Geometry check sheet. Reference: the model listing, model coordinates, mm. A direction names the side the tool comes from. Give positions to 0.01 mm unless a question says otherwise; leave off trailing zeros. Order: outer loops, then holes, each group sorted by start corner. A loop starts at its lowest first (then second) coordinate and runs counter-clockwise, first axis right, second up. Notation, with made-up numbers: M -20,-37.5 L -14,-37.5 A23 ccw -14,-23.5 Z; hole C -38.75,40.5 d11. An arc over 180 degrees is marked long. Answer as CSV lines item,"result".
from build123d import *

# Parameters (mm, degrees)
SKETCH4_R           = 6
BOSS_EXTRUDE3_DEPTH = 1
SKETCH5_R           = 5
SKETCH5_R_2         = 4
BOSS_EXTRUDE4_DEPTH = 4.75
CUT_EXTRUDE3_START  = -3
SKETCH9_R           = 4
CUT_EXTRUDE3_DEPTH  = 3
CUT_EXTRUDE7_DEPTH  = 10
CUT_EXTRUDE8_DEPTH  = 10
CUT_EXTRUDE10_START = -6
CUT_EXTRUDE10_DEPTH = 6
SKETCH14_R          = 2.4
CUT_EXTRUDE11_DEPTH = 6


with BuildPart() as part:
    # Sketch4 → Boss-Extrude3 (new body)
    with BuildSketch(Plane(origin=(0, 0, 0), x_dir=(1, 0, 0), z_dir=(0, 1, 0))):
        with Locations(Location((0, 0, 0), (0, 0, 270))):
            Circle(SKETCH4_R)
    extrude(amount=BOSS_EXTRUDE3_DEPTH)

    # Sketch5 → Boss-Extrude4 (add)
    with BuildSketch(Plane(origin=(0, 1, 0), x_dir=(1, 0, 0), z_dir=(0, 1, 0))):
        with Locations(Location((0, 0, 0), (0, 0, 270))):
            Circle(SKETCH5_R)
        with Locations(Location((0, 0, 0), (0, 0, 270))):
            Circle(SKETCH5_R_2, mode=Mode.SUBTRACT)
    extrude(amount=BOSS_EXTRUDE4_DEPTH)

    # Sketch6 → Revolve4 (revolve)
    with BuildSketch(Plane.XY, mode=Mode.PRIVATE) as revolve4_sk:
        Polygon((0, 5.75), (5, 5.75), (6, 7), (0, 7), align=None)
    revolve(revolve4_sk.sketch.rotate(Axis((0, 5.75, 0), (0, 1, 0)), 270), axis=Axis((0, 5.75, 0), (0, 1, 0)))

    # Sketch9 → Cut-Extrude3 (cut)
    with BuildSketch(Plane(origin=(0, 7, 0), x_dir=(1, 0, 0), z_dir=(0, 1, 0)).offset(CUT_EXTRUDE3_START)):
        with Locations(Location((0, 0, 0), (0, 0, 270))):
            Circle(SKETCH9_R)
    extrude(amount=CUT_EXTRUDE3_DEPTH, mode=Mode.SUBTRACT)

    # Sketch11 → Cut-Extrude7 (cut)
    with BuildSketch(Plane.XY):
        Polygon((0, 4.575), (0, 3.375), (1.2, 3.375), (1.6, 3.375), align=None)
        Polygon((-1.2, 3.375), (0, 3.375), (0, 4.575), (-1.6, 3.375), align=None)
        Polygon((0, 2.175), (0, 3.375), (-1.2, 3.375), (-1.6, 3.375), align=None)
        Polygon((1.2, 3.375), (0, 3.375), (0, 2.175), (1.6, 3.375), align=None)
    extrude(amount=CUT_EXTRUDE7_DEPTH, mode=Mode.SUBTRACT)

    # Sketch12 → Cut-Extrude8 (cut)
    with BuildSketch(Plane(origin=(0, 0, 0), x_dir=(0, 0, -1), z_dir=(1, 0, 0))):
        with BuildLine():
            ThreePointArc((0.6, 3.375), (0.424264069, 3.799264069), (0, 3.975))
            Line((0, 3.975), (0, 2.775))
            ThreePointArc((0, 2.775), (0.424264069, 2.950735931), (0.6, 3.375))
        make_face()
        with BuildLine():
            Line((0, 2.775), (0, 3.975))
            ThreePointArc((0, 3.975), (-0.6, 3.375), (0, 2.775))
        make_face()
    extrude(amount=CUT_EXTRUDE8_DEPTH, mode=Mode.SUBTRACT)

    # Sketch13 → Cut-Extrude10 (cut)
    with BuildSketch(Plane(origin=(0, 7, 0), x_dir=(1, 0, 0), z_dir=(0, 1, 0)).offset(CUT_EXTRUDE10_START)):
        with BuildLine():
            Line((-4.779206309, -3.627559381), (-3.72991173, -1.444907777))
            ThreePointArc((-3.72991173, -1.444907777), (-3.947043415, 0.648728201), (-3.071224525, 2.562728998))
            Line((-3.071224525, 2.562728998), (-4.606836788, 3.844093497))
            ThreePointArc((-4.606836788, 3.844093497), (-5.99840399, 0.138381967), (-4.779206309, -3.627559381))
        make_face()
    extrude(amount=CUT_EXTRUDE10_DEPTH, mode=Mode.SUBTRACT)

    # Sketch14 → Cut-Extrude11 (cut)
    with BuildSketch(Plane(origin=(0, 1, 0), x_dir=(1, 0, 0), z_dir=(0, 1, 0))):
        with Locations(Location((0, 0, 0), (0, 0, 270))):
            Circle(SKETCH14_R)
    extrude(amount=-CUT_EXTRUDE11_DEPTH, mode=Mode.SUBTRACT)


solid = part.part
(1) Gauge pin test, flat ends, axial feed: P1, Ø7, axis at x = 0, z = 0, coming from the +Y side; P2, Ø1.5, axis at x = 0.5, y = 4, coming from the -Z side; P3, Ø2, axis at x = 2.5, y = 1, coming from the +Z side. Record the tip position at first contact, or that the pin passes through.
The answers:
P1,"stops at y = 1"
P2,"stops at z = -5"
P3,"stops at z = 5.81"
(2) Tool access check on faces 1 (the face through (-3.49, 3.96, -2.91)), 2 (the face through (-3, 1, 0)), 3 (the face through (1.802, 0.493, 5.723)). Record the directions out of +Z, -Z, +X, -X, +Y, -Y that give a thin tool (end or side, any length) a straight path to the whole face; none if there is none.
The answers:
face 1,"-X, +Y"
face 2,"none"
face 3,"+Y, -Y"
(3) Section check A-A on x = 0.5. State how many separate pieces and enclosed holes the cut face has, then the cut area to 3 significant figures.
The answers:
separate pieces,"3"
enclosed holes,"0"
area,"18.9 mm2"
(4) Draft check along Y on faces 4 (the face through (3, 7, -3)), 5 (the face through (0, 0, 3)), 6 (the face through (-0.811, 2.783, 4.324)). Enter one of: +Y half, -Y half, draft (parallel to the pull), parting line (faces both ways), or undercut.
The answers:
face 4,"+Y half"
face 5,"-Y half"
face 6,"undercut"
(5) Material ranges on line 1 (X direction, y = 0.6, z = 0); line 2 (Z direction, x = 0, y = 5); line 3 (Z direction, x = 0, y = 4), recorded low to high.
The answers:
line 1,"x = -6 to -2.4, 2.4 to 6"
line 2,"z = -5 to -4, 4 to 5"
line 3,"z = -5 to -4"
(6) Section check B-B on y = 1.75. Enter the section's corners in (x, z), then the cut area to 3 significant figures.
The answers:
outline,"M -4.28,2.59 L -3.73,1.44 A4 cw long -3.07,-2.56 L -3.84,-3.2 A5 ccw long Z"
area,"23.0 mm2"
